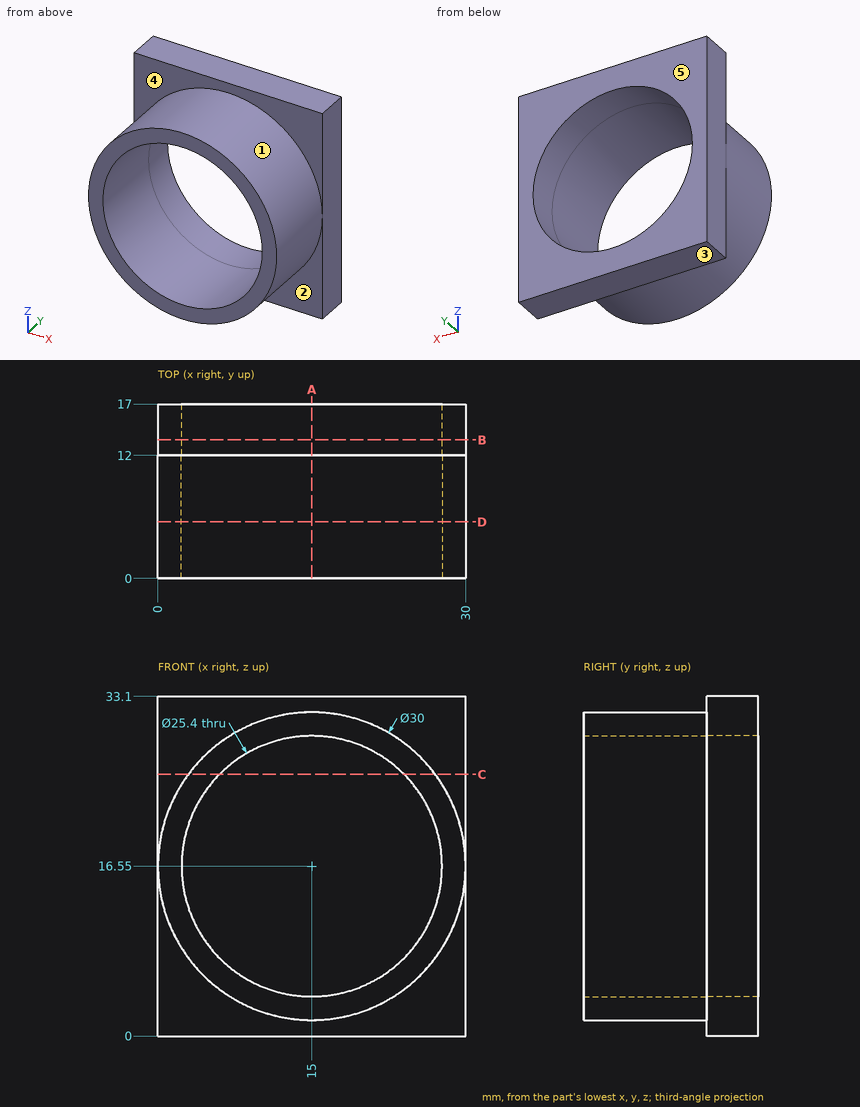
Drawing for the job (mm, zero at the part's lowest x, y, z). A direction names the side the tool comes from. Coordinates: 2 decimals unless noted, no trailing zeros. Order: outer loops, then holes, each group sorted by start corner. A loop starts at its lowest first (then second) coordinate and runs counter-clockwise, first axis right, second up. Notation, with made-up numbers: (-37, -38.75) -> (21, -38.75) arc R20 ccw to (21, -10.75) -> close; hole circle Ø4 at (11.5, 34.25). An arc over 180 degrees is marked (long way). Return JSON: item names as keys, results as strings.
Item 1: Slice it at A-A (x = 15). Write the cut outline in (y, z).
Model answer:
{"outline": "(0, 1.55) -> (12, 1.55) -> (12, 0) -> (17, 0) -> (17, 3.85) -> (0, 3.85) -> close; (0, 29.25) -> (17, 29.25) -> (17, 33.1) -> (12, 33.1) -> (12, 31.55) -> (0, 31.55) -> close"}
Item 2: Slice it at C-C (z = 25.5). Write the cut outline in (x, y).
Model answer:
{"outline": "(0, 12) -> (2.96, 12) -> (2.96, 0) -> (5.99, 0) -> (5.99, 17) -> (0, 17) -> close; (24.01, 0) -> (27.04, 0) -> (27.04, 12) -> (30, 12) -> (30, 17) -> (24.01, 17) -> close"}
Item 3: 3-axis set-ups, long thin cutter, end or side, ignore diameter. For the marked faces 1, 2, 3, 4 and 5: which of +Z, -Z, +X, -X, +Y, -Y reach the whole face in a straight line?
Model answer:
{"face 1": "-Y", "face 2": "-Z, -Y", "face 3": "-Z, +X, -X, +Y, -Y", "face 4": "+Z, -Y", "face 5": "+Z, -Z, +X, -X, +Y"}
Item 4: Slice it at D-D (y = 5.5). Write the cut outline in (x, z).
Model answer:
{"outline": "circle Ø30 at (15, 16.55); hole circle Ø25.4 at (15, 16.55)"}
Item 5: Slice it at B-B (y = 13.5). Write the cut outline in (x, z), then the cut area to 3 significant figures.
Model answer:
{"outline": "(0, 0) -> (30, 0) -> (30, 33.1) -> (0, 33.1) -> close; hole circle Ø25.4 at (15, 16.55)", "area": "486 mm²"}
Item 6: Pin check, flat tip, straight feed: P1, Ø3, axis at y = 5.5, z = 28, coming from the -X side. Stop position of the tip, or through.
Model answer:
{"P1": "stops at x = 3.78"}
Item 7: Wall check: line 1 along Z through (x, y) = (15, 13.35); line 2 along Z through (x, y) = (15, 4.25); line 3 along X through (y, z) = (2, 8). Give the ranges that are in metal, low to high. Write a range as from..to.
Model answer:
{"line 1": "z = 0..3.85, 29.25..33.1", "line 2": "z = 1.55..3.85, 29.25..31.55", "line 3": "x = 2.68..5.61, 24.39..27.32"}
